Work out the finished part from the listing and answer in its coordinate system (mm). A direction names the side the tool comes from. Give positions to 0.01 mm unless a question says otherwise; leave off trailing zeros. Order: outer loops, then holes, each group sorted by start corner. A loop starts at its lowest first (then second) coordinate and runs counter-clockwise, first axis right, second up. Notation, with made-up numbers: (42.25, 73) - (84.25, 73) arc R17 ccw to (84.25, 104) - close; hole circle Ø9 at (55, 47). An arc over 180 degrees is marked (long way). Write each question's results on one line, items separated by ' | '.
from build123d import *

# Parameters (mm, degrees)
PAD_DEPTH       = 13
PAD001_DEPTH    = 13
PAD002_DEPTH    = 13
SKETCH004_R     = 6
POCKET_DEPTH    = 39.001
SKETCH006_W     = 17
SKETCH006_H     = 10
POCKET001_DEPTH = 60


with BuildPart() as part:
    # Sketch001 → Pad (new body)
    with BuildSketch(Plane.XY):
        Polygon((-90.545, 50.821844), (-72.75, 20), (-5, 20), (-5, 35), (0, 35), (0, 33), (50, 33), (50, 22), (0, 22), (0, 20), (80, 20), (80, 0), (-84.297005, 0), (-107.865508, 40.821844), align=None)
    extrude(amount=PAD_DEPTH)

    # Sketch002 (on Face15 of Pad) → Pad001 (join)
    with BuildSketch(Plane(origin=(0, 0, 0), x_dir=(1, 0, 0), z_dir=(0, 0, -1))):
        Polygon((-84.297005, 0), (-72.75, -20), (-77.75, -28.660254), (-89.297005, -8.660254), align=None)
    extrude(amount=PAD001_DEPTH)

    # Sketch003 (on Face12 of Pad001) → Pad002 (join)
    with BuildSketch(Plane(origin=(0, 0, -13), x_dir=(1, 0, 0), z_dir=(0, 0, -1))):
        Polygon((-84.297005, 0), (-107.865508, -40.821844), (-90.545, -50.821844), (-72.75, -20), align=None)
    extrude(amount=PAD002_DEPTH)

    # Sketch004 (on Face26 of Pad002) → Pocket (cut, through all)
    with BuildSketch(Plane(origin=(0, 0, -26), x_dir=(1, 0, 0), z_dir=(0, 0, -1))):
        with Locations((-94.205254, -37.16159)):
            Circle(SKETCH004_R)
    extrude(amount=-POCKET_DEPTH, mode=Mode.SUBTRACT)

    # Sketch006 (on Face21 of Pocket) → Pocket001 (cut)
    with BuildSketch(Plane.YZ.offset(50)):
        with Locations((21, 6.5)):
            Rectangle(SKETCH006_W, SKETCH006_H)
    extrude(amount=-POCKET001_DEPTH, mode=Mode.SUBTRACT)


solid = part.part
1. Straight lines are drawn through the part: line 1 (Z direction, x = 33.5, y = 27); line 2 (Z direction, x = 54, y = 4); line 3 (X direction, y = 42, z = 5). For each, find the intervals that lie inside material, in ascending order. Write a range as [from, to].
Answer list:
line 1: [0, 1.5], [11.5, 13] | line 2: [0, 13] | line 3: [-105.82, -97.75], [-90.66, -85.45]
2. A cutting plane is placed at A-A, the plane z = 6.5. State how many separate pieces and enclosed holes the cut face has, then the cut area to 3 significant figures.
Answer list:
separate pieces: 2 | enclosed holes: 1 | area: 3,640 mm^2
3. A cutting plane is placed at D-D, the plane x = -3. Write down the section's boundary in (y, z), then the cut area to 3 significant figures.
Answer list:
outline: (0, 0) - (35, 0) - (35, 13) - (0, 13) - close; hole (12.5, 1.5) - (29.5, 1.5) - (29.5, 11.5) - (12.5, 11.5) - close | area: 285 mm^2
4. A cutting plane is placed at B-B, the plane y = 27. Write down the section's boundary in (x, z).
Answer list:
outline: (-99.89, -26) - (-76.79, -26) - (-76.79, 13) - (-99.89, 13) - (-99.89, 0) - (-78.71, 0) - (-78.71, -13) - (-99.89, -13) - close; (-5, 0) - (50, 0) - (50, 1.5) - (-5, 1.5) - close; (-5, 11.5) - (50, 11.5) - (50, 13) - (-5, 13) - close
5. Given P1, Ø4, axis at y = 27.5, z = 6, coming from the -X side; P2, Ø0.8, axis at y = 21.5, z = 1, coming from the +X side; P3, Ø1.5, axis at x = -3, z = 4, coming from the +Y side; P4, Ø7, axis at x = -94.21, y = 37.16, coming from the +Z side, each flat-ended and moving along its own axis, determine where each tip first touches the part or whether it passes through.
Answer list:
P1: x = -101.33 | P2: x = 0 | P3: y = 35 | P4: through
6. A tool of negligible diameter and unlimited length cuts with its end or side. For faces 5 (the face through (20, 19, 1.5)), 6 (the face through (-39, 20, 6)), 7 (the face through (-3, 35, 6)), 8 (the face through (-83.443, 18.8, -6.409)), from which of +Z, -Z, +X, -X, +Y, -Y can it reach the whole face along a straight path? Write none if from no direction.
Answer list:
face 5: none | face 6: +Z, -Z, +Y | face 7: +Z, -Z, +X, +Y | face 8: -X, +Y
7. Determine the mould class of faces 1 (the face through (-88.482, 35.359, 6.409)), 2 (the face through (-1, 14, 0)), 3 (the face through (25, 33, 6)), 4 (the face through (-78.443, 10.14, -12.818)) for opening direction Y: +Y half, -Y half, draft (parallel to the pull), parting line (faces both ways), or undercut.
Answer list:
face 1: undercut | face 2: draft | face 3: +Y half | face 4: -Y half
8. A cutting plane is placed at C-C, the plane x = 39.5. Write down the section's boundary in (y, z).
Answer list:
outline: (0, 0) - (20, 0) - (20, 1.5) - (12.5, 1.5) - (12.5, 11.5) - (20, 11.5) - (20, 13) - (0, 13) - close; (22, 0) - (33, 0) - (33, 13) - (22, 13) - (22, 11.5) - (29.5, 11.5) - (29.5, 1.5) - (22, 1.5) - close
